Check sheet for the drawn part. Datum: minimum x, y, z corner. Units: mm. A direction names the side the tool comes from. Give positions to 0.01 mm unless a question says otherwise; leave off trailing zeros. Order: outer loops, then holes, each group sorted by start corner. A loop starts at its lowest first (then second) coordinate and runs counter-clockwise, first axis right, second up.
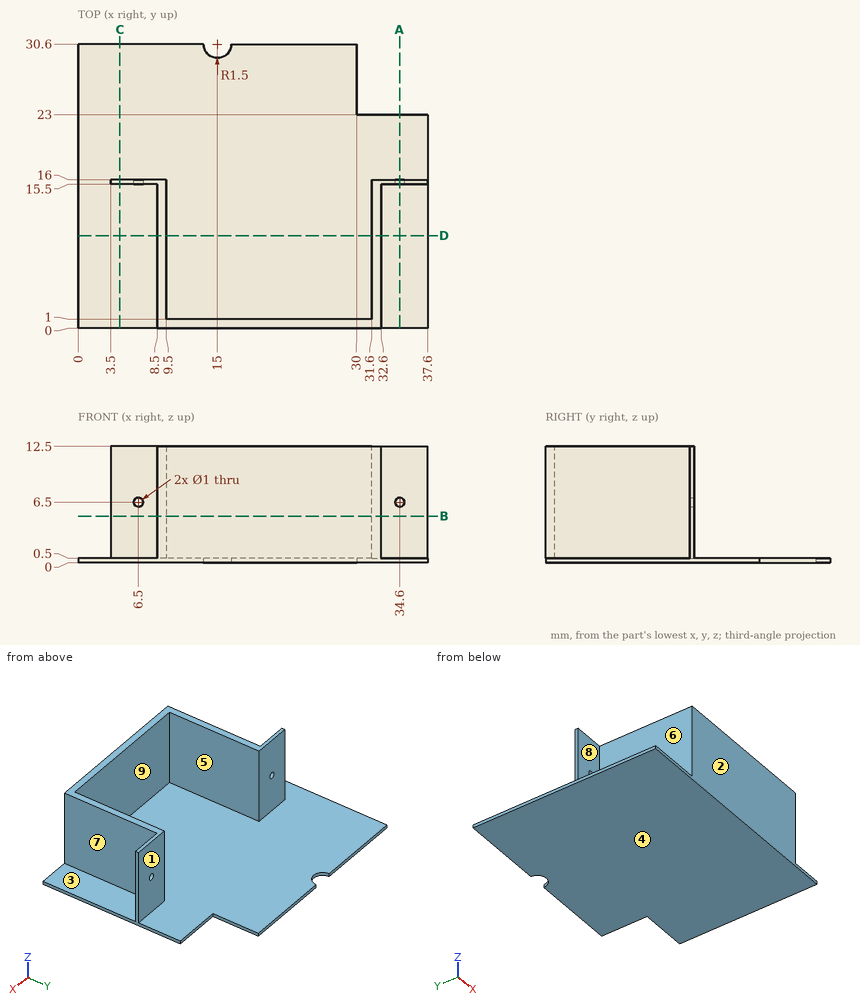
Item 1: Sectioned sample at D-D (y = 10). Enter the section's corners in (x, z).
Reported:
outline: (0, 0) - (37.6, 0) - (37.6, 0.5) - (32.6, 0.5) - (32.6, 12.5) - (31.6, 12.5) - (31.6, 0.5) - (9.5, 0.5) - (9.5, 12.5) - (8.5, 12.5) - (8.5, 0.5) - (0, 0.5) - close
Item 2: Gauge pin test, flat ends, axial feed: pin 1 (6 mm diameter, centred on y = 9.5, z = 9, fed in from -X); pin 2 (15.5 mm diameter, centred on x = 15, y = 23, fed in from +Z); pin 3 (6 mm diameter, centred on x = 16.5, z = 9.5, fed in from +Y); pin 4 (3 mm diameter, centred on y = 22, z = 3, fed in from +X). Record the tip position at first contact, or that the pin passes through.
Reported:
pin 1: stops at x = 8.5
pin 2: stops at z = 0.5
pin 3: stops at y = 1
pin 4: passes through
Item 3: Draft check along X on the marked faces 6, 7, 8 and 9. Enter one of: released by +X, released by -X, zero draft, split by the parting line, or undercut.
Reported:
face 6: released by -X
face 7: released by +X
face 8: zero draft
face 9: undercut
Item 4: Sectioned sample at B-B (z = 5). Enter the section's corners in (x, y).
Reported:
outline: (3.5, 15.5) - (8.5, 15.5) - (8.5, 0) - (32.6, 0) - (32.6, 15.5) - (37.6, 15.5) - (37.6, 16) - (31.6, 16) - (31.6, 1) - (9.5, 1) - (9.5, 16) - (3.5, 16) - close
Item 5: Scan lines: L1, parallel to X at y = 15.6, z = 6.5; L2, parallel to X at y = 3, z = 9; L3, parallel to Z at x = 34.6, y = 15.75. Record each from-to range of solid material in increasing order.
Reported:
L1: x = 3.5 to 6, 7 to 9.5, 31.6 to 34.1, 35.1 to 37.6
L2: x = 8.5 to 9.5, 31.6 to 32.6
L3: z = 0 to 6, 7 to 12.5
Item 6: Sectioned sample at C-C (x = 4.5). Enter the section's corners in (y, z).
Reported:
outline: (0, 0) - (30.6, 0) - (30.6, 0.5) - (16, 0.5) - (16, 12.5) - (15.5, 12.5) - (15.5, 0.5) - (0, 0.5) - close
Item 7: Sectioned sample at A-A (x = 34.6). Enter the section's corners in (y, z).
Reported:
outline: (0, 0) - (23, 0) - (23, 0.5) - (16, 0.5) - (16, 6) - (15.5, 6) - (15.5, 0.5) - (0, 0.5) - close; (15.5, 7) - (16, 7) - (16, 12.5) - (15.5, 12.5) - close
Item 8: Set-up check for the marked faces 1, 2, 3, 4 and 5: record each of +Z, -Z, +X, -X, +Y, -Y from which the full face is reachable in a straight line by a thin tool's end or side.
Reported:
face 1: +Z, +X, -X, +Y
face 2: +Z, -Z, +X, -X, -Y
face 3: +Z, +X, -Y
face 4: -Z, +X, -X, +Y, -Y
face 5: +Z, +Y
